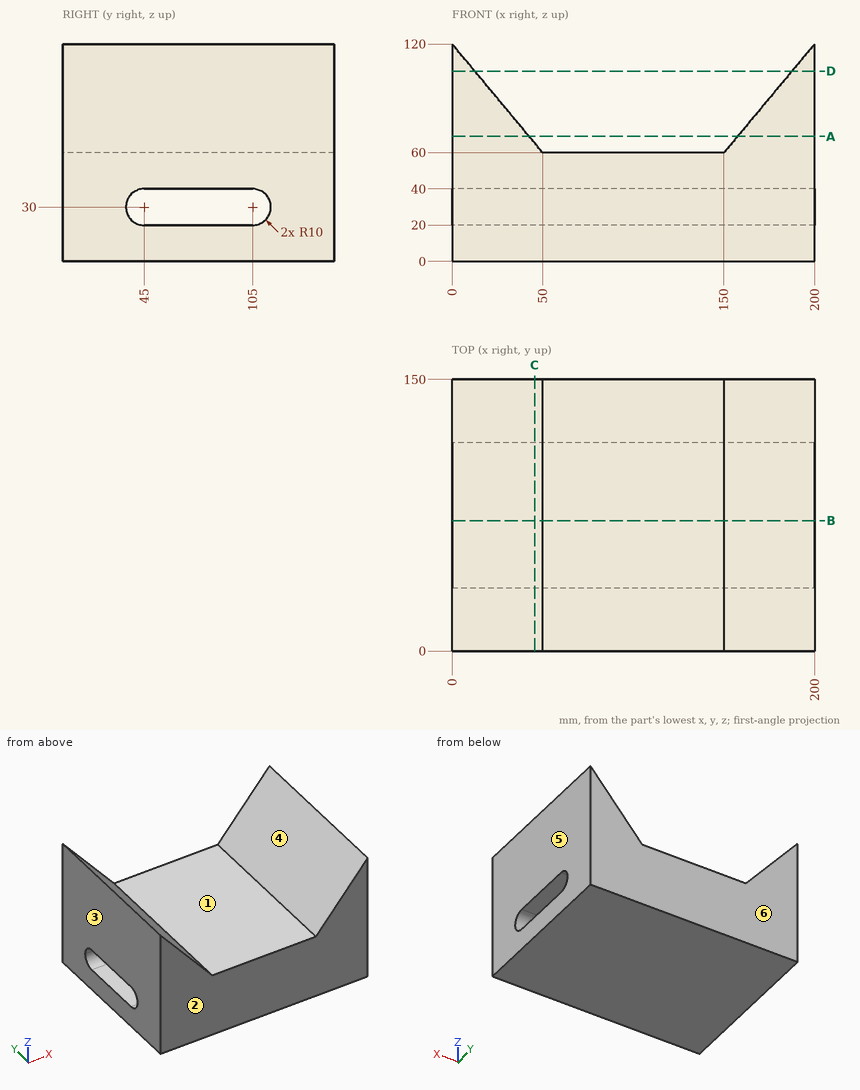
Input: dimensioned drawing with shaded views. Units: mm. Origin: part minimum x, y, z. A direction names the side the tool comes from. Round coordinates to 2 decimals unless told otherwise and drop trailing zeros. Loops run counter-clockwise (first coordinate to the right, second up) from the corner with the lowest first, then second, coordinate; pieces in that order, holes last. Notation, with made-up numbers: M 24.25,14.5 L 54.25,14.5 A31 ccw 54.25,45.5 Z; hole C 28,47.5 d8. An arc over 180 degrees is marked long. Answer in a Markdown table with one row per item. Add a question column.
1. Mould query, pull axis X, two halves, no side actions, for the marked faces 3, 4, 5 and 6. Classes: released by +X, released by -X, zero draft, split by the parting line, or undercut.
2. Section D-D (z = 105). Output: boundary loops of the cut face in (x, y).
3. Section A-A (z = 69). Output: boundary loops of the cut face in (x, y), and give its area (4 significant figures).
4. Ray query, probe 1 along Z at (x, y) = (127, 58); probe 2 along Z at (x, y) = (126, 23); probe 3 along Z at (x, y) = (148.5, 108). Return the intervals inside material, ascending.
5. Section C-C (x = 45.5). Output: boundary loops of the cut face in (y, z).
6. Set-up query: the marked faces 1 and 2. Return all of +Z, -Z, +X, -X, +Y, -Y with unobstructed straight access to the full face (end or side cutting, diameter ignored); none if empty.
7. Section B-B (y = 72). Output: boundary loops of the cut face in (x, z).
Values follow:
| question | item | result |
|---|---|---|
| 1 | face 3 | released by -X |
| 1 | face 4 | undercut |
| 1 | face 5 | released by +X |
| 1 | face 6 | zero draft |
| 2 | outline | M 0,0 L 12.5,0 L 12.5,150 L 0,150 Z; M 187.5,0 L 200,0 L 200,150 L 187.5,150 Z |
| 3 | outline | M 0,0 L 42.5,0 L 42.5,150 L 0,150 Z; M 157.5,0 L 200,0 L 200,150 L 157.5,150 Z |
| 3 | area | 12,750 mm^2 |
| 4 | probe 1 | 0 to 20, 40 to 60 |
| 4 | probe 2 | 0 to 60 |
| 4 | probe 3 | 0 to 20.46, 39.54 to 60 |
| 5 | outline | M 0,0 L 150,0 L 150,65.4 L 0,65.4 Z; hole M 45,20 L 105,20 A10 ccw 105,40 L 45,40 A10 ccw Z |
| 6 | face 1 | +Z, +Y, -Y |
| 6 | face 2 | +Z, -Z, +X, -X, -Y |
| 7 | outline | M 0,0 L 200,0 L 200,20 L 0,20 Z; M 0,40 L 200,40 L 200,120 L 150,60 L 50,60 L 0,120 Z |
